Geometry: final body of the model. Coordinates: model frame, mm. A direction names the side the tool comes from. Give positions to 0.01 mm unless a question says otherwise; leave off trailing zeros. Write each loop counter-clockwise with the first axis right and the second up, starting at its lowest first coordinate (ties: lowest second). Pieces come first, ordered by that corner, then holes. Notation, with made-up numbers: (72, 52.5) -> (82, 52.5) arc R31 ccw to (82, 78.5) -> close; hole circle Ø3 at (27, -11). An arc over 180 degrees is marked (long way). Answer as a JSON object with one key per item and string values.
from build123d import *

# Parameters (mm, degrees)
IZIM1_R                     = 3
IZIM1_R_2                   = 6
Y_KSEKLIK_EKSTR_ZYON1_DEPTH = 10
KES_EKSTR_ZYON1_REACH       = 64.418
KES_EKSTR_ZYON1_END_RADIUS  = 6
IZIM2_R                     = 1.5
SKETCH1_R                   = 5
CUT_EXTRUDE1_DEPTH          = 6


with BuildPart() as part:
    # Çizim1 → Yükseklik-Ekstrüzyon1 (new body)
    with BuildSketch(Plane.XY):
        with BuildLine():
            Line((30, -14), (-25, -14))
            ThreePointArc((-25, -14), (-28.535533906, -12.535533906), (-30, -9))
            Line((-30, -9), (-30, 9))
            ThreePointArc((-30, 9), (-28.535533906, 12.535533906), (-25, 14))
            Line((-25, 14), (30, 14))
            Line((30, 14), (30, -14))
        make_face()
        with Locations((23, 7)):
            Circle(IZIM1_R, mode=Mode.SUBTRACT)
        with Locations((-19, 0)):
            Circle(IZIM1_R_2, mode=Mode.SUBTRACT)
        with Locations((9, -7)):
            Circle(IZIM1_R, mode=Mode.SUBTRACT)
    extrude(amount=Y_KSEKLIK_EKSTR_ZYON1_DEPTH)

    # Kes-Ekstrüzyon1: up to this cylinder (the profile starts outside it)
    kes_ekstr_zyon1_end = Plane(origin=(-19, 0, 5), z_dir=(0, 0, -1)) * Cylinder(KES_EKSTR_ZYON1_END_RADIUS, 141.836, mode=Mode.PRIVATE)
    # Çizim2 → Kes-Ekstrüzyon1 (cut, up to the surface)
    with BuildSketch(Plane.ZY.offset(30), mode=Mode.PRIVATE) as kes_ekstr_zyon1_sk1:
        with Locations((5, 0)):
            Circle(IZIM2_R)
    kes_ekstr_zyon1_tool1 = extrude(kes_ekstr_zyon1_sk1.sketch, amount=-KES_EKSTR_ZYON1_REACH, mode=Mode.PRIVATE) - kes_ekstr_zyon1_end
    add(kes_ekstr_zyon1_tool1.solids().sort_by_distance((-30, 0, 5))[0], mode=Mode.SUBTRACT)

    # Sketch1 → Cut-Extrude1 (cut)
    with BuildSketch(Plane.XY.offset(10)):
        with Locations((9, -7)):
            Circle(SKETCH1_R)
        with Locations((23, 7)):
            Circle(SKETCH1_R)
    extrude(amount=-CUT_EXTRUDE1_DEPTH, mode=Mode.SUBTRACT)


solid = part.part
Q1. Cut plane C-C (z = 5). Return the cut outline in (x, y), and give its area (3 significant figures).
Values:
{"outline": "(-30, -9) arc R5 ccw to (-25, -14) -> (30, -14) -> (30, 14) -> (-25, 14) arc R5 ccw to (-30, 9) -> (-30, 1.5) -> (-24.81, 1.5) arc R6 cw (long way) to (-24.81, -1.5) -> (-30, -1.5) -> close; hole circle Ø10 at (9, -7); hole circle Ø10 at (23, 7)", "area": "1,380 mm²"}
Q2. Material intervals for L1, parallel to X at y = 7, z = 2.05; L2, parallel to Y at x = -19, z = 3.75; L3, parallel to X at y = 1.5, z = 0.75, sorted ascending. Write a range as from..to.
Values:
{"L1": "-30..20, 26..30", "L2": "-14..-6, 6..14", "L3": "-30..-24.81, -13.19..30"}
Q3. Set-up query: faces 5 (the cylindrical face through (-27.441, -0.575, 6.386)), 6 (the flat face through (-30, -2, 5)), 7 (the cylindrical face through (13.77, -5.5, 7.04)). Return all of +Z, -Z, +X, -X, +Y, -Y with unobstructed straight access to the full face (end or side cutting, diameter ignored); none if empty.
Values:
{"face 5": "-X", "face 6": "+Z, -Z, -X, +Y, -Y", "face 7": "+Z"}
Q4. Mould query, pull axis X, two halves, no side actions, for faces 1 (the flat face through (2, 14, 5)), 2 (the flat face through (22.9, 3.7, 4)), 3 (the flat face through (12.3, -6.9, 4)), 4 (the cylindrical face through (-28, -13, 5)). Classes: pulls with the +X half, pulls with the -X half, needs draft (parallel to the pull), parting line crosses it, or undercut.
Values:
{"face 1": "needs draft", "face 2": "undercut", "face 3": "undercut", "face 4": "pulls with the -X half"}
Q5. Cut plane B-B (x = -19). Return the cut outline in (y, z), and give its area (3 significant figures).
Values:
{"outline": "(-14, 0) -> (-6, 0) -> (-6, 10) -> (-14, 10) -> close; (6, 0) -> (14, 0) -> (14, 10) -> (6, 10) -> close", "area": "160 mm²"}
Q6. Cut plane A-A (y = 0). Return the cut outline in (x, z).
Values:
{"outline": "(-30, 0) -> (-25, 0) -> (-25, 3.5) -> (-30, 3.5) -> close; (-30, 6.5) -> (-25, 6.5) -> (-25, 10) -> (-30, 10) -> close; (-13, 0) -> (30, 0) -> (30, 10) -> (-13, 10) -> close"}
Q7. First-contact query: P1, Ø1.8, axis at y = 0, z = 5, coming from the -X side; P2, Ø3, axis at x = 22.5, y = 4.5, coming from the +Z side; P3, Ø1.5, axis at x = -19.5, y = -3.5, coming from the -Z side. Flat tips, straight axial feed; report the tip coordinate or a pass-through.
Values:
{"P1": "x = -13.07", "P2": "z = 4", "P3": "through"}
Q8. Cut plane D-D (y = -7). Return the cut outline in (x, z).
Values:
{"outline": "(-30, 0) -> (6, 0) -> (6, 4) -> (4, 4) -> (4, 10) -> (-30, 10) -> close; (12, 0) -> (30, 0) -> (30, 10) -> (14, 10) -> (14, 4) -> (12, 4) -> close"}
